```python
from build123d import *

# Parameters (mm, degrees)
F5_DEPTH = 3
F7_DEPTH = 17
F8_W     = 15
F8_H     = 4
F8_W_2   = 3.5
F8_H_2   = 10.5
F9_DEPTH = 2.001


with BuildPart() as f3:
    # F0 (on Top) → F3 section 0
    with BuildSketch(Plane.XY):
        Polygon((-4, 67), (-4, -4), (46, -4), (46, 19.3431457505), (50.5, 23.8431457505), (50.5, 42.1568542495), (46, 46.6568542495), (46, 67), align=None)
    # F2 (on offset) → F3 section 1
    with BuildSketch(Plane.XY.offset(16)):
        Polygon((0, 63), (0, 0), (42, 0), (42, 21), (46.5, 25.5), (46.5, 40.5), (42, 45), (42, 63), align=None)
    loft()

    # F4 (on face) → F5 (join)
    with BuildSketch(Plane(origin=(0, 0, 0), x_dir=(1, 0, 0), z_dir=(0, 0, -1))):
        Polygon((46, 4), (-4, 4), (-4, -67), (46, -67), (46, -46.6568542495), (50.5, -42.1568542495), (50.5, -23.8431457505), (46, -19.3431457505), align=None)
    extrude(amount=F5_DEPTH)

    # F6 (on face) → F7 (cut)
    with BuildSketch(Plane.XY.offset(16)):
        with BuildLine():
            Line((38.95, 61), (3.05, 61))
            ThreePointArc((3.05, 61), (2.4843145751, 60.7656854249), (2.25, 60.2))
            Line((2.25, 60.2), (2.25, 2.8))
            ThreePointArc((2.25, 2.8), (2.4843145751, 2.2343145751), (3.05, 2))
            Line((3.05, 2), (38.95, 2))
            ThreePointArc((38.95, 2), (39.5156854249, 2.2343145751), (39.75, 2.8))
            Line((39.75, 2.8), (39.75, 21.1686291501))
            ThreePointArc((39.75, 21.1686291501), (39.810896374, 21.474775896), (39.9843145751, 21.7343145751))
            Line((39.9843145751, 21.7343145751), (44.5156854249, 26.2656854249))
            ThreePointArc((44.5156854249, 26.2656854249), (44.689103626, 26.525224104), (44.75, 26.8313708499))
            Line((44.75, 26.8313708499), (44.75, 39.6686291501))
            ThreePointArc((44.75, 39.6686291501), (44.689103626, 39.974775896), (44.5156854249, 40.2343145751))
            Line((44.5156854249, 40.2343145751), (39.9843145751, 44.7656854249))
            ThreePointArc((39.9843145751, 44.7656854249), (39.810896374, 45.025224104), (39.75, 45.3313708499))
            Line((39.75, 45.3313708499), (39.75, 60.2))
            ThreePointArc((39.75, 60.2), (39.5156854249, 60.7656854249), (38.95, 61))
        make_face()
    extrude(amount=-F7_DEPTH, mode=Mode.SUBTRACT)

    # F8 (on face) → F9 (cut, through all)
    with BuildSketch(Plane.XY.offset(-1)):
        with Locations((18.75, 55.5)):
            Rectangle(F8_W, F8_H)
        with Locations((41, 33.75)):
            Rectangle(F8_W_2, F8_H_2)
    extrude(amount=-F9_DEPTH, mode=Mode.SUBTRACT)


solid = f3.part
```
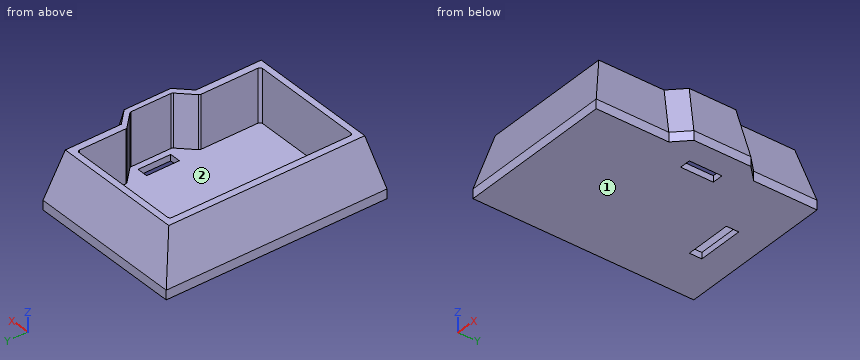
Geometry: final body of the model. Coordinates: model frame, mm. Face numbers are marked on the shaded views. Round coordinates to 2 decimals unless told otherwise and drop trailing zeros. Use one line per item in the form item = value. Start each with the question number.
1. Pin query (flat end, axial travel): pin 1 Ø4 at (x, z) = (8, 4) entering from -Y; pin 2 Ø2.5 at (y, z) = (59, -1.5) entering from +X; pin 3 Ø21 at (x, y) = (14.5, 21) entering from +Z; pin 4 Ø5 at (x, y) = (43, 9.5) entering from +Z. Return the tip coordinate at first contact, or that it passes through.
2. Line query: probe 1 along X at (y, z) = (44, 0); probe 2 along Y at (x, z) = (34, 13.75); probe 3 along Z at (x, y) = (37, 50.5). Output: solid intervals per line, ascending.
3. Draft query along X for the marked faces 1 and 2. Return one class per face: pulls with the +X half, pulls with the -X half, needs draft (parallel to the pull), parting line crosses it, or undercut.
Solution:
q1.pin_1 = -3.5
q1.pin_2 = 46
q1.pin_3 = -1
q1.pin_4 = 16
q2.probe_1 = -4 to 2.25, 40.75 to 48.66
q2.probe_2 = -0.56 to 2, 61 to 63.56
q2.probe_3 = -3 to -1
q3.face_1 = needs draft
q3.face_2 = undercut
